from build123d import *

# Parameters (mm, degrees)
F1_DEPTH = 5
F2_T     = -1


with BuildPart() as f1:
    # F0 (on Top) → F1 (new body)
    with BuildSketch(Plane.XY):
        with BuildLine():
            ThreePointArc((-10, 60), (-95.3553390593, 95.3553390593), (-60, 10))
            Line((-60, 10), (-60, -10))
            ThreePointArc((-60, -10), (-95.3553390593, -95.3553390593), (-10, -60))
            Line((-10, -60), (10, -60))
            ThreePointArc((10, -60), (95.3553390593, -95.3553390593), (60, -10))
            Line((60, -10), (60, 10))
            ThreePointArc((60, 10), (95.3553390593, 95.3553390593), (10, 60))
            Line((10, 60), (-10, 60))
        make_face()
        with BuildLine():
            Line((-50, -60), (-12.5, -60))
            ThreePointArc((-12.5, -60), (-93.5875721064, -93.5875721064), (-60, -12.5))
            Line((-60, -12.5), (-60, -50))
            ThreePointArc((-60, -50), (-67.0710678119, -67.0710678119), (-50, -60))
        make_face(mode=Mode.SUBTRACT)
        with BuildLine():
            ThreePointArc((-55, -12.7638909308), (-26.4124278936, -26.4124278936), (-12.7638909308, -55))
            Line((-12.7638909308, -55), (-51.3397459622, -55))
            ThreePointArc((-51.3397459622, -55), (-52.9289321881, -52.9289321881), (-55, -51.3397459622))
            Line((-55, -51.3397459622), (-55, -12.7638909308))
        make_face(mode=Mode.SUBTRACT)
        with BuildLine():
            Line((12.5, -60), (50, -60))
            ThreePointArc((50, -60), (67.0710678119, -67.0710678119), (60, -50))
            Line((60, -50), (60, -12.5))
            ThreePointArc((60, -12.5), (93.5875721064, -93.5875721064), (12.5, -60))
        make_face(mode=Mode.SUBTRACT)
        with BuildLine():
            Line((-16.6987298108, -35), (16.6987298108, -35))
            ThreePointArc((16.6987298108, -35), (12.4121286857, -44.6574283846), (10.2506281447, -55))
            Line((10.2506281447, -55), (-10.2506281447, -55))
            ThreePointArc((-10.2506281447, -55), (-12.4121286857, -44.6574283846), (-16.6987298108, -35))
        make_face(mode=Mode.SUBTRACT)
        with BuildLine():
            ThreePointArc((12.7638909308, -55), (26.4124278936, -26.4124278936), (55, -12.7638909308))
            Line((55, -12.7638909308), (55, -51.3397459622))
            ThreePointArc((55, -51.3397459622), (52.9289321881, -52.9289321881), (51.3397459622, -55))
            Line((51.3397459622, -55), (12.7638909308, -55))
        make_face(mode=Mode.SUBTRACT)
        with BuildLine():
            Line((55, 10.2506281447), (55, -10.2506281447))
            ThreePointArc((55, -10.2506281447), (38.8033952288, -14.7153011915), (25, -24.2928578573))
            Line((25, -24.2928578573), (25, 24.2928578573))
            ThreePointArc((25, 24.2928578573), (38.8033952288, 14.7153011915), (55, 10.2506281447))
        make_face(mode=Mode.SUBTRACT)
        with BuildLine():
            Line((-25, 24.2928578573), (-25, -24.2928578573))
            ThreePointArc((-25, -24.2928578573), (-38.8033952288, -14.7153011915), (-55, -10.2506281447))
            Line((-55, -10.2506281447), (-55, 10.2506281447))
            ThreePointArc((-55, 10.2506281447), (-38.8033952288, 14.7153011915), (-25, 24.2928578573))
        make_face(mode=Mode.SUBTRACT)
        with BuildLine():
            ThreePointArc((-12.7638909308, 55), (-26.4124278936, 26.4124278936), (-55, 12.7638909308))
            Line((-55, 12.7638909308), (-55, 51.3397459622))
            ThreePointArc((-55, 51.3397459622), (-52.9289321881, 52.9289321881), (-51.3397459622, 55))
            Line((-51.3397459622, 55), (-12.7638909308, 55))
        make_face(mode=Mode.SUBTRACT)
        with BuildLine():
            Line((16.6987298108, 35), (-16.6987298108, 35))
            ThreePointArc((-16.6987298108, 35), (-12.4121286857, 44.6574283846), (-10.2506281447, 55))
            Line((-10.2506281447, 55), (10.2506281447, 55))
            ThreePointArc((10.2506281447, 55), (12.4121286857, 44.6574283846), (16.6987298108, 35))
        make_face(mode=Mode.SUBTRACT)
        with BuildLine():
            ThreePointArc((-50, 60), (-67.0710678119, 67.0710678119), (-60, 50))
            Line((-60, 50), (-60, 12.5))
            ThreePointArc((-60, 12.5), (-93.5875721064, 93.5875721064), (-12.5, 60))
            Line((-12.5, 60), (-50, 60))
        make_face(mode=Mode.SUBTRACT)
        with BuildLine():
            ThreePointArc((55, 12.7638909308), (26.4124278936, 26.4124278936), (12.7638909308, 55))
            Line((12.7638909308, 55), (51.3397459622, 55))
            ThreePointArc((51.3397459622, 55), (52.9289321881, 52.9289321881), (55, 51.3397459622))
            Line((55, 51.3397459622), (55, 12.7638909308))
        make_face(mode=Mode.SUBTRACT)
        with BuildLine():
            ThreePointArc((60, 50), (67.0710678119, 67.0710678119), (50, 60))
            Line((50, 60), (12.5, 60))
            ThreePointArc((12.5, 60), (93.5875721064, 93.5875721064), (60, 12.5))
            Line((60, 12.5), (60, 50))
        make_face(mode=Mode.SUBTRACT)
    extrude(amount=F1_DEPTH)

    # F2
    f2_openings = [f1.faces().sort_by_distance(p)[0] for p in [
        (0, 0, 5),
    ]]
    offset(amount=F2_T, openings=f2_openings, kind=Kind.INTERSECTION)


solid = f1.part
Check sheet for the modelled part. Datum: model origin and axes. Units: mm. A direction names the side the tool comes from. Give positions to 0.01 mm unless a question says otherwise; leave off trailing zeros. Answer as a JSON object with one key per item and string values. Group by question number.
Q1. Go/stop test with flat-tipped pins: P1, Ø3, axis at x = 37, z = 3, coming from the -Y side; P2, Ø1.5, axis at x = -25.5, z = 2, coming from the -Y side; P3, Ø2.5, axis at x = 4, z = 1.5, coming from the -Y side. Record where each tip stops, or that it passes through.
Q2. Release check for a two-part mould opening along Y. For faces 1 (the flat face through (-24.7, 0.1, 5)), 2 (the cylindrical face through (66.834, -67.3, 2.465)), 3 (the flat face through (0, -60, 2)) record: released by +Y, released by -Y, zero draft, split by the parting line, or undercut.
Q3. Material ranges on line 1 along X through (y, z) = (1, 0.9); line 2 along X through (y, z) = (7, 3.5); line 3 along Y through (x, z) = (36, 0.35), recorded low to high. Write a range as [from, to].
Q4. Cross-section at A-A on y = -79. Give the number of separate pieces and of enclosed holes in the cut face, then the cut area to 3 significant figures.
Q5. Access from +Z, -Z, +X, -X, +Y, -Y to the whole of each face (thin tool, end or side, straight path). Record for faces 4 (the flat face through (60, 31, 2)), 5 (the cylindrical face through (25.37, -26.044, 2.972)).
Evaluation:
{
 "1": {"P1": "stops at y = -105.14", "P2": "stops at y = -96.89", "P3": "stops at y = -60"},
 "2": {"face 1": "zero draft", "face 2": "undercut", "face 3": "released by -Y"},
 "3": {"line 1": "x = [-60, -55], [-25, 25], [55, 60]", "line 2": "x = [-60, -59], [-56, -55], [-25, -24], [24, 25], [55, 56], [59, 60]", "line 3": "y = [-103.86, -100.99], [-60, -55], [-19.01, -16.14], [16.14, 19.01], [55, 60], [100.99, 103.86]"},
 "4": {"separate pieces": "4", "enclosed holes": "0", "area": "45.6 mm2"},
 "5": {"face 4": "+Z, -Z", "face 5": "+Z"}
}
